```python
from build123d import *

# Parameters (mm, degrees)
SKIZZE3_R                            = 5.5
SKIZZE3_R_2                          = 4.5
AUFSATZ_LINEAR_AUSTRAGEN1_DEPTH      = 578.1
SKIZZE5_OUTSIDE_W                    = 164.65
SKIZZE5_OUTSIDE_H                    = 696.15
SKIZZE5_OUTSIDE_W_2                  = 45.6
SKIZZE5_OUTSIDE_H_2                  = 24
SKIZZE5_OUTSIDE_R                    = 2
SCHNITT_LINEAR_AUSTRAGEN2_DEPTH      = 9.85
SCHNITT_LINEAR_AUSTRAGEN2_DEPTH_BACK = 9.85
SKETCH2_R                            = 1.25
CUT_EXTRUDE1_DEPTH                   = 6


with BuildPart() as part:
    # Skizze3 → Aufsatz-Linear austragen1 (new body)
    with BuildSketch(Plane(origin=(0, 0, 0), x_dir=(1, 0, 0), z_dir=(0, 1, 0))):
        Polygon((-12.6, -8.85), (-12.6, 8.85), (19, 8.85), (19, 6.85), (34, 6.85), (34, 3.85), (22, 3.85), (22, -3.85), (34, -3.85), (34, -6.85), (19, -6.85), (19, -8.85), align=None)
        Circle(SKIZZE3_R, mode=Mode.SUBTRACT)
        with Locations((14, 0)):
            Circle(SKIZZE3_R_2, mode=Mode.SUBTRACT)
    extrude(amount=AUFSATZ_LINEAR_AUSTRAGEN1_DEPTH)

    # Skizze5 outside → Schnitt-Linear austragen2 (cut, two sides)
    with BuildSketch(Plane.XY) as schnitt_linear_austragen2_sk:
        with Locations((10.7, 289.05)):
            Rectangle(SKIZZE5_OUTSIDE_W, SKIZZE5_OUTSIDE_H)
        with Locations((11.2, 566.1)):
            Rectangle(SKIZZE5_OUTSIDE_W_2, SKIZZE5_OUTSIDE_H_2, mode=Mode.SUBTRACT)
        with Locations((29, 566.1)):
            Circle(SKIZZE5_OUTSIDE_R)
    extrude(amount=SCHNITT_LINEAR_AUSTRAGEN2_DEPTH, mode=Mode.SUBTRACT)
    extrude(schnitt_linear_austragen2_sk.sketch, amount=-SCHNITT_LINEAR_AUSTRAGEN2_DEPTH_BACK, mode=Mode.SUBTRACT)

    # Sketch2 → Cut-Extrude1 (cut)
    with BuildSketch(Plane(origin=(0, 578.1, 0), x_dir=(1, 0, 0), z_dir=(0, 1, 0))):
        with Locations((-7.155344001, 5.459034001)):
            Circle(SKETCH2_R)
        with Locations((7.155344001, -5.459034001)):
            Circle(SKETCH2_R)
    extrude(amount=-CUT_EXTRUDE1_DEPTH, mode=Mode.SUBTRACT)


solid = part.part
```
Geometry: final body of the model. Coordinates: model frame, mm. A direction names the side the tool comes from. Round coordinates to 2 decimals unless told otherwise and drop trailing zeros. Loops run counter-clockwise (first coordinate to the right, second up) from the corner with the lowest first, then second, coordinate; pieces in that order, holes last. Notation, with made-up numbers: (79, -22.5) -> (122, -22.5) arc R10 ccw to (122, -10.5) -> close; hole circle Ø9 at (37.25, 69.5). An arc over 180 degrees is marked (long way). Use one line per item in the form item = value.
Item 1: Cut plane C-C on y = 556.25. Output: boundary loops of the cut face in (x, z), then the cut area to 3 significant figures.
Evaluation:
outline = (-11.6, -8.85) -> (19, -8.85) -> (19, -6.85) -> (34, -6.85) -> (34, -3.85) -> (22, -3.85) -> (22, 3.85) -> (34, 3.85) -> (34, 6.85) -> (19, 6.85) -> (19, 8.85) -> (-11.6, 8.85) -> close; hole circle Ø11 at (0, 0); hole circle Ø9 at (14, 0)
area = 496 mm2
Item 2: Material intervals for probe 1 along X at (y, z) = (565.5, 0); probe 2 along Z at (x, y) = (14, 561); probe 3 along Z at (x, y) = (0, 560.5), sorted ascending.
Evaluation:
probe_1 = -11.6 to -5.5, 5.5 to 9.5, 18.5 to 22
probe_2 = -8.85 to -4.5, 4.5 to 8.85
probe_3 = -8.85 to -5.5, 5.5 to 8.85
Item 3: Draft query along X for faces 1 (the flat face through (22, 566, 0)), 2 (the flat face through (26.6, 565.9, 3.85)), 3 (the cylindrical face through (18.292, 565.932, -1.352)). Return one class per face: released by +X, released by -X, zero draft, split by the parting line, or undercut.
Evaluation:
face_1 = released by +X
face_2 = zero draft
face_3 = undercut
Item 4: Cut plane B-B on x = 0. Output: boundary loops of the cut face in (y, z), then the cut area to 3 significant figures.
Evaluation:
outline = (554.1, -8.85) -> (578.1, -8.85) -> (578.1, -5.5) -> (554.1, -5.5) -> close; (554.1, 5.5) -> (578.1, 5.5) -> (578.1, 8.85) -> (554.1, 8.85) -> close
area = 161 mm2
Item 5: Contact query for flat-ended pins moving along their axis: pin 1 Ø13 at (x, y) = (27, 565) entering from +Z; pin 2 Ø2 at (x, z) = (-7.16, -5.46) entering from +Y; pin 3 Ø9.5 at (x, y) = (29.5, 562.5) entering from -Z; pin 4 Ø3 at (x, z) = (-7.5, -5.5) entering from +Y. Output: stop coordinate, or through.
Evaluation:
pin_1 = 6.85
pin_2 = 572.1
pin_3 = -6.85
pin_4 = 578.1
Item 6: Cut plane D-D on z = -6.25. Output: boundary loops of the cut face in (x, y).
Evaluation:
outline = (-11.6, 554.1) -> (34, 554.1) -> (34, 578.1) -> (-6.19, 578.1) -> (-6.19, 572.1) -> (-8.12, 572.1) -> (-8.12, 578.1) -> (-11.6, 578.1) -> close; hole circle Ø4 at (29, 566.1)
Item 7: Cut plane A-A on y = 566.1. Output: boundary loops of the cut face in (x, z).
Evaluation:
outline = (-11.6, -8.85) -> (19, -8.85) -> (19, -6.85) -> (27, -6.85) -> (27, -3.85) -> (22, -3.85) -> (22, 3.85) -> (27, 3.85) -> (27, 6.85) -> (19, 6.85) -> (19, 8.85) -> (-11.6, 8.85) -> close; (31, -6.85) -> (34, -6.85) -> (34, -3.85) -> (31, -3.85) -> close; (31, 3.85) -> (34, 3.85) -> (34, 6.85) -> (31, 6.85) -> close; hole circle Ø11 at (0, 0); hole circle Ø9 at (14, 0)
Item 8: Access query for faces 4 (the flat face through (19, 566, 8)), 5 (the flat face through (26, 566, -6.85)), 6 (the flat face through (7, 572.1, 5)). Directions: +Z, -Z, +X, -X, +Y, -Y. A direction counts if a zero-diameter tool reaches every point of the face in a straight line with its end or side. Return the directions, or none.
Evaluation:
face_4 = +Z, +X, +Y, -Y
face_5 = -Z, +X, +Y, -Y
face_6 = +Y
